The model under review builds one solid part; all positions refer to its coordinate system, in mm. A direction names the side the tool comes from. Give positions to 0.01 mm unless a question says otherwise; leave off trailing zeros. Order: outer loops, then holes, each group sorted by start corner. A loop starts at its lowest first (then second) coordinate and runs counter-clockwise, first axis right, second up. Notation, with made-up numbers: (39.5, -32.75) - (62.5, -32.75) arc R14 ccw to (62.5, -8.75) - close; hole circle Ø6 at (-29.75, 42.5). An arc over 180 degrees is marked (long way). Use CSV: the item, a comma, the result in double quotes. Start each with the question number.
1. Take a section at C-C, the plane z = -1. State the section outline as (x, y) points.
2. Draft analysis for pull direction Y (two halves, no side actions). For faces 5 (the flat face through (3.302, 24.965, 4.508)), 6 (the flat face through (15.3, -20, 4.5)), 7 (the flat face through (-22.189, 4.827, 4.508)), state which applies: released by +Y, released by -Y, zero draft, split by the parting line, or undercut.
3. Take a section at A-A, the plane x = 3. State the section outline as (y, z) points, then the cut area to 3 significant figures.
4. Take a section at B-B, the plane y = -15.5. State the section outline as (x, z) points.
5. Take a section at D-D, the plane y = 6.5. State the section outline as (x, z) points, then the cut area to 3 significant figures.
6. For pin 1 (4 mm diameter, centred on y = -15.5, z = -0.5, fed in from +X); pin 2 (1.5 mm diameter, centred on x = -16.5, z = 9, fed in from +Y); pin 3 (2 mm diameter, centred on x = 9.5, y = 8, fed in from +Z), all flat-tipped, find the tip position at first contact; note any pin that passes through.
7. To check wall thickness, follow line 1 (Y direction, x = 0, z = -1.2); line 2 (X direction, y = 18, z = 1.5); line 3 (Z direction, x = 6, y = 16.5). State the ranges of each line that lie inside material, in increasing order. Write a range as [from, to].
8. Machinability: for faces 1 (the flat face through (4.827, 22.189, 4.508)), 2 (the flat face through (-22.262, -4.815, 4.508)), 3 (the flat face through (15.3, -16.87, 4.51)), 4 (the flat face through (4.815, -22.262, 4.508)), which of the approach directions +Z, -Z, +X, -X, +Y, -Y give a long, thin tool a straight path to every point of the face, cutting with its end or side? Answer none if there is none.
```python
from build123d import *

# Parameters (mm, degrees)
F0_R     = 10.16
F1_DEPTH = 9.144
F0_R_2   = 3.81
F2_DEPTH = 10.922
F3_DEPTH = 1.778


with BuildPart() as f1:
    # F0 (on Top) → F1 (new body)
    with BuildSketch(Plane.XY):
        Polygon((-2.192223, 25.111405), (-4.383126, 24.822963), (-5.259222, 19.627621), (-8.616823, 23.68837), (-10.658424, 22.842703), (-10.16, 17.597653), (-14.454226, 20.650987), (-16.207359, 19.305753), (-14.368424, 14.368424), (-19.306565, 16.206318), (-20.651826, 14.453159), (-17.597653, 10.16), (-22.843211, 10.65718), (-23.688878, 8.615604), (-19.627621, 5.259197), (-24.823141, 4.381805), (-25.111583, 2.190902), (-20.32, 0), (-25.111405, -2.192198), (-24.822963, -4.3831), (-19.627621, -5.259197), (-23.68837, -8.616823), (-22.842703, -10.658399), (-17.597653, -10.16), (-20.651013, -14.4542), (-19.305753, -16.207359), (-14.368424, -14.368399), (-16.206318, -19.306565), (-14.453159, -20.6518), (-10.16, -17.597628), (-10.65718, -22.843211), (-8.615604, -23.688853), (-5.259222, -19.627596), (-4.381805, -24.823115), (-2.190902, -25.111558), (0, -20.32), (2.192198, -25.11138), (4.3831, -24.822937), (5.259197, -19.627596), (8.616823, -23.688345), (10.658399, -22.842703), (10.16, -17.597628), (14.4542, -20.650987), (16.207359, -19.305753), (14.368399, -14.368399), (19.306565, -16.206292), (20.6518, -14.453159), (17.597628, -10.16), (22.843211, -10.65718), (23.688853, -8.615578), (19.627596, -5.259197), (24.823115, -4.381779), (25.111558, -2.190902), (20.32, 0), (25.11138, 2.192223), (24.822937, 4.383126), (19.627596, 5.259197), (23.688345, 8.616823), (22.842677, 10.658424), (17.597628, 10.16), (20.650987, 14.4542), (19.305753, 16.207359), (14.368399, 14.368424), (16.206292, 19.306565), (14.453133, 20.6518), (10.16, 17.597653), (10.65718, 22.843211), (8.615578, 23.688878), (5.259197, 19.627621), (4.381779, 24.823141), (2.190877, 25.111558), (0, 20.32), align=None)
        Circle(F0_R, mode=Mode.SUBTRACT)
    extrude(amount=F1_DEPTH)

    # F0 (on Top) → F2 (join)
    with BuildSketch(Plane.XY):
        Circle(F0_R)
        Circle(F0_R_2, mode=Mode.SUBTRACT)
    extrude(amount=F2_DEPTH)

    # F0 (on Top) → F3 (join)
    with BuildSketch(Plane.XY):
        Circle(F0_R)
        Circle(F0_R_2, mode=Mode.SUBTRACT)
    extrude(amount=-F3_DEPTH)


solid = f1.part
```
Determined:
1,outline,"circle Ø20.32 at (0, 0); hole circle Ø7.62 at (0, 0)"
2,face 5,"released by +Y"
2,face 6,"released by -Y"
2,face 7,"undercut"
3,outline,"(-25.01, 0) - (-9.71, 0) - (-9.71, -1.78) - (-2.35, -1.78) - (-2.35, 10.92) - (-9.71, 10.92) - (-9.71, 9.14) - (-25.01, 9.14) - close; (2.35, -1.78) - (9.71, -1.78) - (9.71, 0) - (25.01, 0) - (25.01, 9.14) - (9.71, 9.14) - (9.71, 10.92) - (2.35, 10.92) - close"
3,area,"467 mm²"
4,outline,"(-19.85, 0) - (-17.41, 0) - (-17.41, 9.14) - (-19.85, 9.14) - close; (-14.79, 0) - (14.79, 0) - (14.79, 9.14) - (-14.79, 9.14) - close; (17.41, 0) - (19.85, 0) - (19.85, 9.14) - (17.41, 9.14) - close"
5,outline,"(-21.13, 0) - (-7.81, 0) - (-7.81, -1.78) - (7.81, -1.78) - (7.81, 0) - (21.13, 0) - (21.13, 9.14) - (7.81, 9.14) - (7.81, 10.92) - (-7.81, 10.92) - (-7.81, 9.14) - (-21.13, 9.14) - close"
5,area,"442 mm²"
6,pin 1,"stops at x = 20.65"
6,pin 2,"stops at y = 19.66"
6,pin 3,"stops at z = 9.14"
7,line 1,"y = [-10.16, -3.81], [3.81, 10.16]"
7,line 2,"x = [-15.72, -10.73], [-10.2, 10.2], [10.73, 15.72]"
7,line 3,"z = [0, 9.14]"
8,face 1,"+Z, -Z, +Y"
8,face 2,"+Z, -Z, -X"
8,face 3,"+Z, -Z"
8,face 4,"+Z, -Z, -Y"
